```python
from build123d import *

# Parameters (mm, degrees)
SKETCH1_W           = 140
SKETCH1_H           = 44
BOSS_EXTRUDE1_DEPTH = 56
FILLET1_R           = 8
SKETCH2_R           = 0.907650606
BOSS_EXTRUDE2_DEPTH = 1


with BuildPart() as part:
    # Sketch1 → Boss-Extrude1 (new body)
    with BuildSketch(Plane(origin=(0, 0, 0), x_dir=(1, 0, 0), z_dir=(0, 1, 0))):
        Rectangle(SKETCH1_W, SKETCH1_H)
    extrude(amount=BOSS_EXTRUDE1_DEPTH)

    # Fillet1
    fillet1_edges = [part.edges().sort_by_distance(p)[0] for p in [
        (-70, 56, 0),
        (0, 56, 22),
        (70, 56, 0),
        (0, 0, 22),
        (-70, 0, 0),
        (0, 0, -22),
        (70, 0, 0),
        (0, 56, -22),
        (70, 28, 22),
        (-70, 28, 22),
        (-70, 28, -22),
        (70, 28, -22),
    ]]
    fillet(fillet1_edges, radius=FILLET1_R)

    # Sketch2 → Boss-Extrude2 (add)
    with BuildSketch(Plane(origin=(0, 0, -22), x_dir=(-1, 0, 0), z_dir=(0, 0, -1))):
        with Locations(Location((0, 28, 0), (0, 0, 180))):
            Circle(SKETCH2_R)
    extrude(amount=BOSS_EXTRUDE2_DEPTH)


solid = part.part
```
Part model, mm, in its own coordinate system. Round coordinates to 2 decimals unless told otherwise and drop trailing zeros. Loops run counter-clockwise (first coordinate to the right, second up) from the corner with the lowest first, then second, coordinate; pieces in that order, holes last.
Item 1: Drop a flat-ended pin along its axis: P1, Ø12, axis at x = 17.5, y = 26, coming from the -Z side. Give the stop position or say it passes through.
Item 2: Drill centre lines: line 1 (Z direction, x = -36.5, y = 24); line 2 (Y direction, x = 62.5, z = 13.5); line 3 (Z direction, x = 23, y = 49). Where is each one in solid material? Low to high.
Item 3: Cut at A-A, the plane y = 36. Give the cut face in (x, z).
Item 4: Cut at B-B, the plane x = 56.5. Give the cut face in (y, z).
A:
1. P1: stops at z = -22
2. line 1: z = -22 to 22
2. line 2: y = 0.02 to 55.98
2. line 3: z = -21.94 to 21.94
3. outline: (-70, -14) arc R8 ccw to (-62, -22) - (62, -22) arc R8 ccw to (70, -14) - (70, 14) arc R8 ccw to (62, 22) - (-62, 22) arc R8 ccw to (-70, 14) - close
4. outline: (0, -14) arc R8 ccw to (8, -22) - (48, -22) arc R8 ccw to (56, -14) - (56, 14) arc R8 ccw to (48, 22) - (8, 22) arc R8 ccw to (0, 14) - close
